Could you check a few things on this model? Use its own coordinates, in mm. A direction names the side the tool comes from. Give positions to 0.01 mm unless a question says otherwise; leave off trailing zeros. Write each loop counter-clockwise with the first axis right and the second up, starting at its lowest first coordinate (ties: lowest second). Pieces come first, ordered by that corner, then holes. Notation, with made-up numbers: (-22, 14) - (23, 14) arc R27 ccw to (23, 52) - close; hole circle Ø3 at (-12, 35.25). An arc over 180 degrees is marked (long way). Answer as a JSON object with one key per item and string values. Group by question number.
```python
from build123d import *

# Parameters (mm, degrees)
SKETCH1_R           = 1.7
BOSS_EXTRUDE1_DEPTH = 3
SKETCH2_W           = 19.2
SKETCH2_H           = 24
BOSS_EXTRUDE2_DEPTH = 22.752
SKETCH3_R           = 7.5
CUT_EXTRUDE1_DEPTH  = 41.290513821


with BuildPart() as part:
    # Sketch1 → Boss-Extrude1 (new body)
    with BuildSketch(Plane(origin=(0, 0, 0), x_dir=(1, 0, 0), z_dir=(0, 1, 0))):
        Polygon((-9.6, 5), (-9.6, 12), (9.6, 12), (9.6, 5), (19.6, 5), (19.6, -5), (9.6, -5), (9.6, -12), (-9.6, -12), (-9.6, -5), (-19.6, -5), (-19.6, 5), align=None)
        with Locations(Location((-14.6, 0, 0), (0, 0, 270))):
            Circle(SKETCH1_R, mode=Mode.SUBTRACT)
        with Locations(Location((14.6, 0, 0), (0, 0, 270))):
            Circle(SKETCH1_R, mode=Mode.SUBTRACT)
    extrude(amount=BOSS_EXTRUDE1_DEPTH)

    # Sketch2 → Boss-Extrude2 (add)
    with BuildSketch(Plane(origin=(0, 3, 0), x_dir=(1, 0, 0), z_dir=(0, 1, 0))):
        Rectangle(SKETCH2_W, SKETCH2_H)
    extrude(amount=BOSS_EXTRUDE2_DEPTH)

    # Sketch3 → Cut-Extrude1 (cut, through all)
    with BuildSketch(Plane.XY.offset(12)):
        with Locations((0, 9.5)):
            Circle(SKETCH3_R)
    extrude(amount=-CUT_EXTRUDE1_DEPTH, mode=Mode.SUBTRACT)


solid = part.part
```
(1) If we mould it in two halves opening along Z, with no side actions, what happens to faces 1 (the cylindrical face through (12.94, 1.48, -0.37)), 2 (the flat face through (0, 18, -12)), 3 (the flat face through (9.6, 13, 0)), 4 (the flat face through (15, 1, 5))? For each: +Z half, -Z half, draft (parallel to the pull), parting line (faces both ways), or undercut.
(2) I want a section at A-A, the plane y = 9.5. Please give me the cut outline in (x, z), and give its area (3 significant figures).
(3) I want a section at B-B, the plane z = 0. Please give me the cut outline in (x, y), and give its area (3 significant figures).
(4) Will these pins go through, and if not, where does the flat tip stop? P1, Ø3, axis at y = 7, z = -1.5, coming from the -X side; P2, Ø2.5, axis at x = 15.5, y = 1.5, coming from the +Z side; P3, Ø8, axis at x = -16, z = 0, coming from the +Y side.
(5) I need wall thicknesses on L1, parallel to X at y = 1.15, z = 0; L2, parallel to Y at x = 0, z = 3; L3, parallel to Y at x = 17, z = 3. Which ranges of each line are inside material? Lowest first, please.
(6) For faces 5 (the flat face through (-15, 1, -5)), 6 (the flat face through (-15, 1, 5)), 7 (the flat face through (12, 3, 0)), 8 (the flat face through (15, 1, -5)), which set-ups out of +Z, -Z, +X, -X, +Y, -Y let a thin tool reach every point of the face, with its end or its side?
(7) I want a section at C-C, the plane x = 0. Please give me the cut outline in (y, z).
(8) I want a section at D-D, the plane z = 10. Please give me the cut outline in (x, y).
Entries:
{
 "1": {"face 1": "undercut", "face 2": "-Z half", "face 3": "draft", "face 4": "+Z half"},
 "2": {"outline": "(-9.6, -12) - (-7.5, -12) - (-7.5, 12) - (-9.6, 12) - close; (7.5, -12) - (9.6, -12) - (9.6, 12) - (7.5, 12) - close", "area": "101 mm^2"},
 "3": {"outline": "(-19.6, 0) - (-16.3, 0) - (-16.3, 3) - (-19.6, 3) - close; (-12.9, 0) - (12.9, 0) - (12.9, 3) - (9.6, 3) - (9.6, 25.75) - (-9.6, 25.75) - (-9.6, 3) - (-12.9, 3) - close; (16.3, 0) - (19.6, 0) - (19.6, 3) - (16.3, 3) - close; hole circle Ø15 at (0, 9.5)", "area": "357 mm^2"},
 "4": {"P1": "x = -9.6", "P2": "z = 5", "P3": "y = 3"},
 "5": {"L1": "-19.6 to -16.3, -12.9 to 12.9, 16.3 to 19.6", "L2": "0 to 2, 17 to 25.75", "L3": "0 to 3"},
 "6": {"face 5": "-Z, -X, +Y, -Y", "face 6": "+Z, -X, +Y, -Y", "face 7": "+Z, -Z, +X, +Y", "face 8": "-Z, +X, +Y, -Y"},
 "7": {"outline": "(0, -12) - (2, -12) - (2, 12) - (0, 12) - close; (17, -12) - (25.75, -12) - (25.75, 12) - (17, 12) - close"},
 "8": {"outline": "(-9.6, 0) - (9.6, 0) - (9.6, 25.75) - (-9.6, 25.75) - close; hole circle Ø15 at (0, 9.5)"}
}
